Check sheet for the drawn part. Datum: minimum x, y, z corner. Units: mm. Round coordinates to 2 decimals unless told otherwise and drop trailing zeros. Write each loop counter-clockwise with the first axis right and the second up, starting at its lowest first coordinate (ties: lowest second). Pieces come first, ordered by that corner, then holes. Notation, with made-up numbers: (46.5, 51.25) - (79.5, 51.25) arc R30 cw to (79.5, 80.25) - close; hole circle Ø2 at (81.5, 74). An arc over 180 degrees is marked (long way). Answer as a JSON object with one key per item and string values.
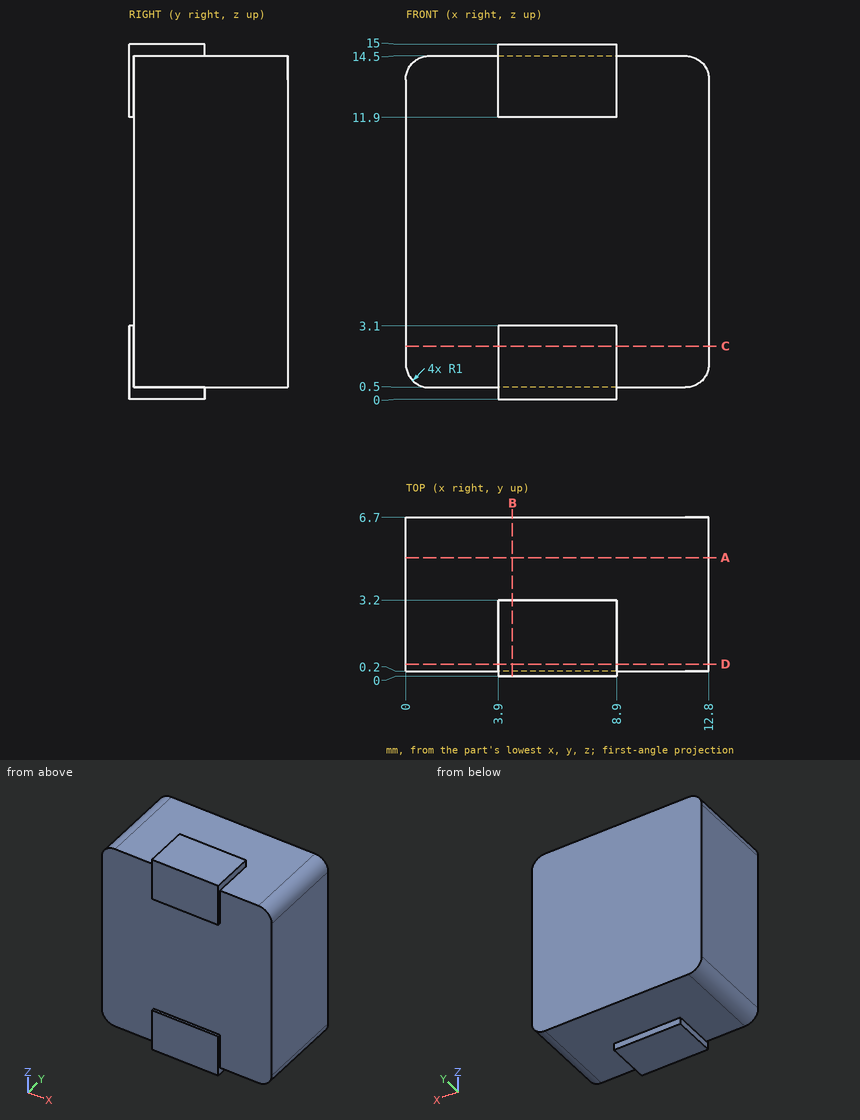
1. Material ranges on probe 1 along Z at (x, y) = (2.75, 1.75); probe 2 along Y at (x, z) = (1.25, 9); probe 3 along X at (y, z) = (1, 1.25), recorded low to high. Write a range as from..to.
Completed:
{"probe 1": "z = 0.5..14.5", "probe 2": "y = 0.2..6.7", "probe 3": "x = 0.03..12.77"}
2. Cross-section at D-D (y = 0.5). Record the boundary of the cut face in (x, z).
Completed:
{"outline": "(0, 1.5) arc R1 ccw to (1, 0.5) - (3.9, 0.5) - (3.9, 0) - (8.9, 0) - (8.9, 0.5) - (11.8, 0.5) arc R1 ccw to (12.8, 1.5) - (12.8, 13.5) arc R1 ccw to (11.8, 14.5) - (8.9, 14.5) - (8.9, 15) - (3.9, 15) - (3.9, 14.5) - (1, 14.5) arc R1 ccw to (0, 13.5) - close"}
3. Cross-section at C-C (z = 2.25). Record the boundary of the cut face in (x, y), plus the area to 3 significant figures.
Completed:
{"outline": "(0, 0.2) - (3.9, 0.2) - (3.9, 0) - (8.9, 0) - (8.9, 0.2) - (12.8, 0.2) - (12.8, 6.7) - (0, 6.7) - close", "area": "84.2 mm^2"}
4. Go/stop test with flat-tipped pins: pin 1 (3 mm diameter, centred on x = 4, z = 7.5, fed in from -Y); pin 2 (4 mm diameter, centred on x = 3.5, y = 1.5, fed in from +Z); pin 3 (0.6 mm diameter, centred on x = 7.5, z = 15, fed in from +Y); pin 4 (1.5 mm diameter, centred on x = 11.5, y = 2.5, fed in from +Z). Record where each tip stops, or that it passes through.
Completed:
{"pin 1": "stops at y = 0.2", "pin 2": "stops at z = 15", "pin 3": "stops at y = 3.2", "pin 4": "stops at z = 14.5"}
5. Cross-section at B-B (x = 4.5). Record the boundary of the cut face in (y, z).
Completed:
{"outline": "(0, 0) - (3.2, 0) - (3.2, 0.5) - (6.7, 0.5) - (6.7, 14.5) - (3.2, 14.5) - (3.2, 15) - (0, 15) - (0, 11.9) - (0.2, 11.9) - (0.2, 3.1) - (0, 3.1) - close"}
6. Cross-section at A-A (y = 5). Record the boundary of the cut face in (x, z), plus the area to 3 significant figures.
Completed:
{"outline": "(0, 1.5) arc R1 ccw to (1, 0.5) - (11.8, 0.5) arc R1 ccw to (12.8, 1.5) - (12.8, 13.5) arc R1 ccw to (11.8, 14.5) - (1, 14.5) arc R1 ccw to (0, 13.5) - close", "area": "178 mm^2"}
